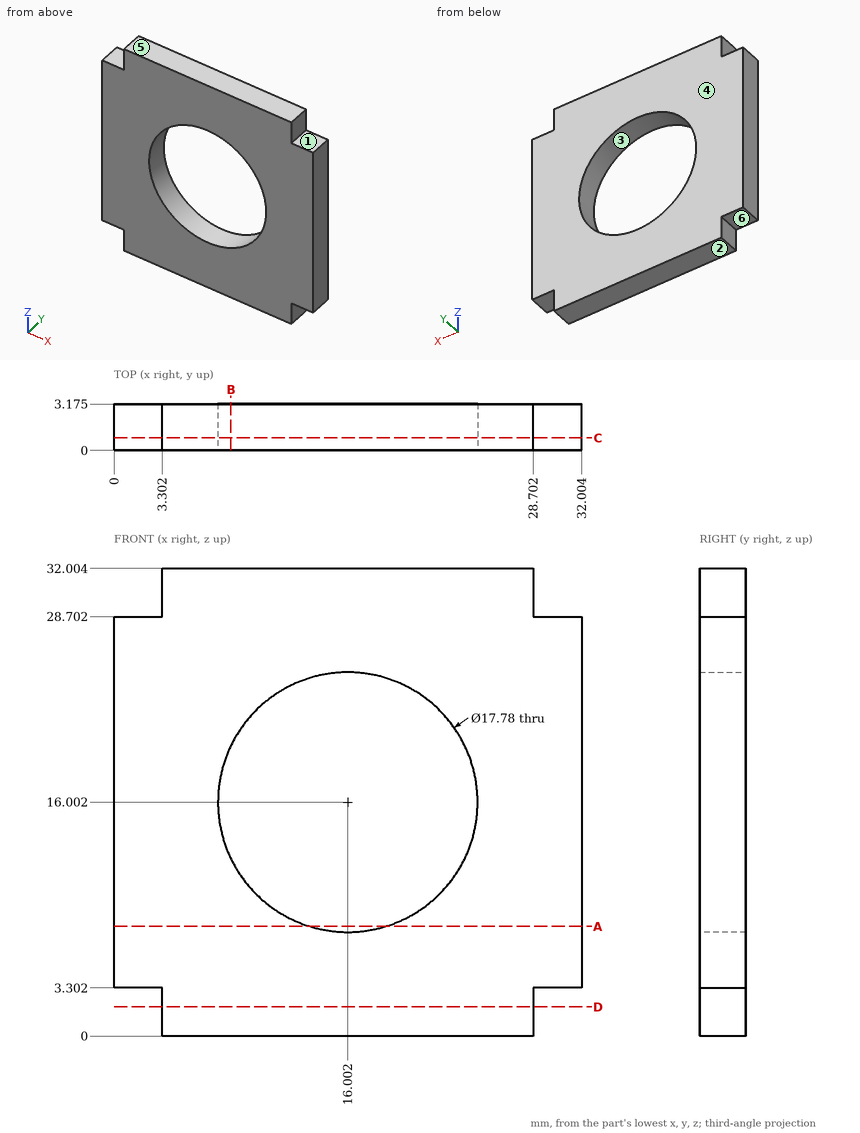
Geometry check sheet. Reference: drawing and pictorial views, mm from the part's lowest x, y, z. A direction names the side the tool comes from. Coordinates: 2 decimals unless noted, no trailing zeros. Order: outer loops, then holes, each group sorted by start corner. A loop starts at its lowest first (then second) coordinate and runs counter-clockwise, first axis right, second up. Notation, with made-up numbers: (47.25, 76.5) -> (59.25, 76.5) arc R27 cw to (59.25, 113.5) -> close; hole circle Ø4 at (-2, -4). An arc over 180 degrees is marked (long way). Write item = value, one per line. Start each with the question number.
1) Cross-section at C-C (y = 0.85). Enter the section's corners in (x, z), then the cut area to 3 significant figures.
2) Cross-section at A-A (z = 7.5). Enter the section's corners in (x, y) (3 decimals), then the cut area to 3 significant figures.
3) Go/stop test with flat-tipped pins: P1, Ø1.6, axis at x = 31, y = 2, coming from the +Z side; P2, Ø1, axis at y = 2, z = 2, coming from the -X side; P3, Ø1, axis at x = 29.5, y = 1.5, coming from the -Z side. Record where each tip stops, or that it passes through.
4) Access from +Z, -Z, +X, -X, +Y, -Y to the whole of each face (thin tool, end or side, straight path). Record for the marked faces 5 and 6.
5) Cross-section at B-B (x = 8). Enter the section's corners in (y, z) (3 decimals).
6) Mould release check, pull along Z, two halves, no side actions. Record for the marked faces 1, 2, 3 and 4: +Z half, -Z half, draft (parallel to the pull), parting line (faces both ways), or undercut.
7) Cross-section at D-D (z = 2). Enter the section's corners in (x, y) (3 decimals).
8) Material ranges on L1, parallel to Z at x = 9.5, y = 2.95; L2, parallel to Z at x = 31.5, y = 0.45; L3, parallel to X at y = 0.4, z = 19, recorded low to high.
Ans:
q1.outline = (0, 3.3) -> (3.3, 3.3) -> (3.3, 0) -> (28.7, 0) -> (28.7, 3.3) -> (32, 3.3) -> (32, 28.7) -> (28.7, 28.7) -> (28.7, 32) -> (3.3, 32) -> (3.3, 28.7) -> (0, 28.7) -> close; hole circle Ø17.78 at (16, 16)
q1.area = 732 mm²
q2.outline = (0, 0) -> (13.404, 0) -> (13.404, 3.175) -> (0, 3.175) -> close; (18.6, 0) -> (32.004, 0) -> (32.004, 3.175) -> (18.6, 3.175) -> close
q2.area = 85.1 mm²
q3.P1 = 28.7
q3.P2 = 3.3
q3.P3 = 3.3
q4.face_5 = +Z, +X, -X, +Y, -Y
q4.face_6 = -Z, -X, +Y, -Y
q5.outline = (0, 0) -> (3.175, 0) -> (3.175, 12.129) -> (0, 12.129) -> close; (0, 19.875) -> (3.175, 19.875) -> (3.175, 32.004) -> (0, 32.004) -> close
q6.face_1 = +Z half
q6.face_2 = -Z half
q6.face_3 = undercut
q6.face_4 = draft
q7.outline = (3.302, 0) -> (28.702, 0) -> (28.702, 3.175) -> (3.302, 3.175) -> close
q8.L1 = 0 to 9.94, 22.06 to 32
q8.L2 = 3.3 to 28.7
q8.L3 = 0 to 7.63, 24.37 to 32
